Autodesk Inventor part; units mm, degrees
ref_plane "YZ Plane" through (0, 0, 0) normal (1, 0, 0) x (0, 1, 0)
ref_plane "XZ Plane" through (0, 0, 0) normal (0, 1, 0) x (-1, 0, 0)
ref_plane "XY Plane" through (0, 0, 0) normal (0, 0, 1) x (1, 0, 0)
sketch "Sketch1" plane through (0, 0, 0) normal (1, 0, 0) x (0, 1, 0)
  line L0 (33.0238, 38.0801) -> (-116.9762, 38.0801)
  line L1 (-116.9762, 38.0801) -> (-116.9762, 31.188)
  line L2 (-116.9762, 31.188) -> (33.0238, 31.188)
  line L3 (33.0238, 31.188) -> (33.0238, 38.0801)
  point P0 (0, 0)
  dimension "d0" = 150
extrude "Extrusion1" add sketch "Sketch1" along normal blind 2
sketch "Sketch2" plane through (2, 0, 0) normal (1, 0, 0) x (0, 0, -1)
  line L0 (-38.0801, -116.9762) -> (-31.188, -116.9762)
  line L1 (-34.4927, -40.2559) -> (-32.849, -40.2559)
  line L2 (-32.849, -40.2559) -> (-32.849, -116.9762)
  line L3 (-32.849, -116.9762) -> (-34.4927, -116.9762)
  line L4 (-34.4927, -116.9762) -> (-34.4927, -40.2559)
  point P0 (0, 0)
extrude "Extrusion2" add sketch "Sketch2" along normal blind 2
fillet "Fillet1" radius 1 1 edges at (4, -40.2559, 33.6708)
properties part number "lock4"
Design review of the part built by this model. Coordinates are the model's own, in mm. Give positions to 0.01 mm unless a question says otherwise; leave off trailing zeros. Write each loop counter-clockwise with the first axis right and the second up, starting at its lowest first coordinate (ties: lowest second). Pieces come first, ordered by that corner, then holes. Notation, with made-up numbers: M -29.75,88.5 L 9.25,88.5 A31 ccw 9.25,115.5 Z; hole C -5.75,84.5 d10. An arc over 180 degrees is marked long. Return JSON: item names as keys, results as strings. Group by question number.
Item 1: Take a section at B-B (z = 36). Give the boundary of the cut face in (x, y).
Item 2: Wall thickness on line 1 along X through (y, z) = (-67, 36.75); line 2 along Z through (x, y) = (3.15, -93); line 3 along Y through (x, z) = (2.6, 33.75): over which ranges is each line inside the solid? List them lowest first.
Item 3: Take a section at A-A (y = -53.5). Give the boundary of the cut face in (x, z).
Item 4: Take a section at C-C (y = 19). Give the boundary of the cut face in (x, z), plus the area to 3 significant figures.
Item 5: Clearance check with flat-ended pins moving along their axes: pin 1 Ø0.6 at (x, y) = (3, -72.5) entering from -Z; pin 2 Ø3 at (y, z) = (-5.5, 36.5) entering from -X; pin 3 Ø0.5 at (x, z) = (2.5, 33.5) entering from +Y; pin 4 Ø0.6 at (x, y) = (3.5, -78) entering from +Z. State where each tip first meets the part, or that it passes through.
Return value:
{
 "1": {"outline": "M 0,-116.98 L 2,-116.98 L 2,33.02 L 0,33.02 Z"},
 "2": {"line 1": "x = 0 to 2", "line 2": "z = 32.85 to 34.49", "line 3": "y = -116.98 to -40.26"},
 "3": {"outline": "M 0,31.19 L 2,31.19 L 2,32.85 L 4,32.85 L 4,34.49 L 2,34.49 L 2,38.08 L 0,38.08 Z"},
 "4": {"outline": "M 0,31.19 L 2,31.19 L 2,38.08 L 0,38.08 Z", "area": "13.8 mm2"},
 "5": {"pin 1": "stops at z = 32.85", "pin 2": "stops at x = 0", "pin 3": "stops at y = -40.26", "pin 4": "stops at z = 34.49"}
}
